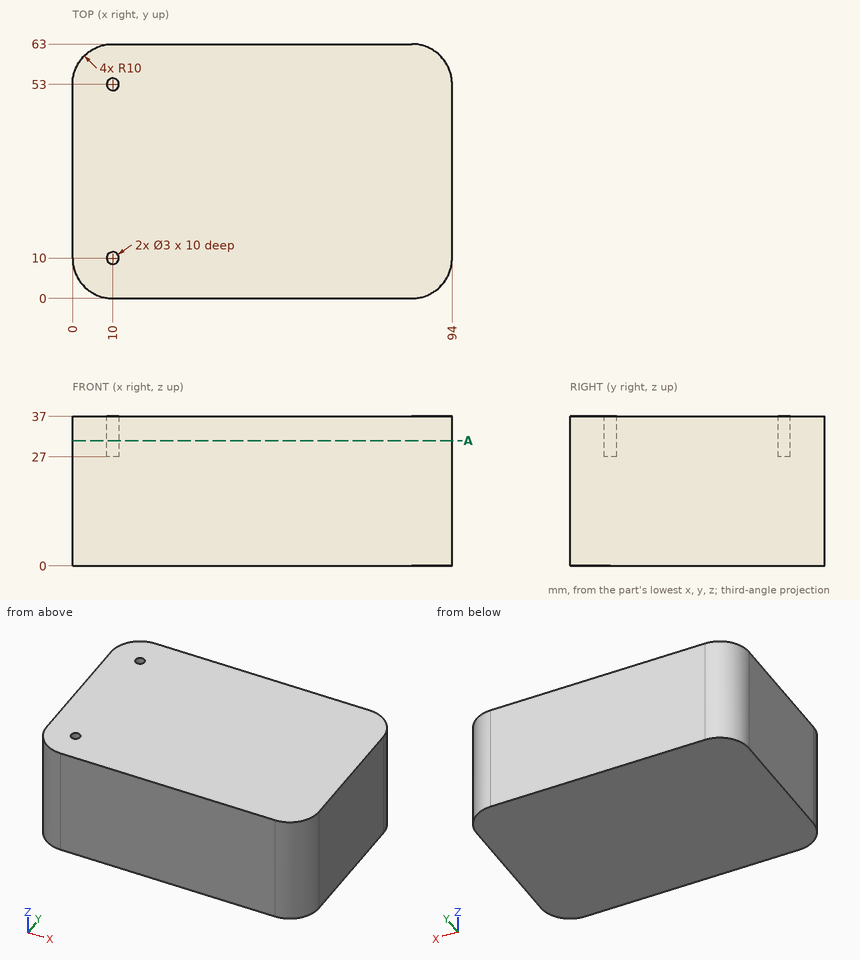
Source: three-view drawing plus pictorial views. Frame: mm from the lowest corner of the part. Round coordinates to 2 decimals unless told otherwise and drop trailing zeros. Loops run counter-clockwise (first coordinate to the right, second up) from the corner with the lowest first, then second, coordinate; pieces in that order, holes last.
Q1. First-contact query: P1, Ø1, axis at y = 9, z = 17, coming from the -X side; P2, Ø12, axis at x = 61, z = 12, coming from the -Y side; P3, Ø0.9, axis at x = 10.5, y = 10, coming from the +Z side. Flat tips, straight axial feed; report the tip coordinate or a pass-through.
Q2. Ray query, line 1 (Y direction, x = 10, z = 30.5); line 2 (X direction, y = 54.5, z = 6); line 3 (Y direction, x = 85, z = 34.5). Return the intervals inside material, ascending.
Q3. Section A-A, the plane z = 31. Return loops of the section in (x, y), plus the area to 3 significant figures.
Solutions:
1. P1: stops at x = 0.01
1. P2: stops at y = 0
1. P3: stops at z = 27
2. line 1: y = 0 to 8.5, 11.5 to 51.5, 54.5 to 63
2. line 2: x = 0.11 to 93.89
2. line 3: y = 0.05 to 62.95
3. outline: (0, 10) arc R10 ccw to (10, 0) - (84, 0) arc R10 ccw to (94, 10) - (94, 53) arc R10 ccw to (84, 63) - (10, 63) arc R10 ccw to (0, 53) - close; hole circle Ø3 at (10, 10); hole circle Ø3 at (10, 53)
3. area: 5,820 mm2
